```python
from build123d import *

# Parameters (mm, degrees)
EXTRUDE_1_DEPTH        = 25
HOLE_WIZARD_M4_1_D     = 3.3
HOLE_WIZARD_M4_1_DEPTH = 20
HOLE_WIZARD_M4_1_TIP   = 0.991420021
SKETCH_5_R             = 2
EXTRUDE_2_DEPTH        = 6


# Read off the part's stored shape, not the designer's step: M4 机械螺纹 螺柱1
with BuildPart() as part:
    # 草图1 → 凸台-拉伸1 (new body)
    with BuildSketch(Plane.XY):
        Polygon((-3.464101615, 0), (-1.732050808, -3), (1.732050808, -3), (3.464101615, 0), (1.732050808, 3), (-1.732050808, 3), align=None)
    extrude(amount=EXTRUDE_1_DEPTH)

    # M4 螺纹孔1
    with Locations(Plane.XY.offset(25)):
        with Locations((0, 0)):
            Hole(HOLE_WIZARD_M4_1_D / 2, depth=HOLE_WIZARD_M4_1_DEPTH)
            with Locations((0, 0, -(HOLE_WIZARD_M4_1_DEPTH + HOLE_WIZARD_M4_1_TIP / 2))):  # 118° drill point
                Cone(0, HOLE_WIZARD_M4_1_D / 2, HOLE_WIZARD_M4_1_TIP, mode=Mode.SUBTRACT)

    # 草图5 → 凸台-拉伸2 (add)
    with BuildSketch(Plane(origin=(0, 0, 0), x_dir=(-1, 0, 0), z_dir=(0, 0, -1))):
        Circle(SKETCH_5_R)
    extrude(amount=EXTRUDE_2_DEPTH)

    # M4 机械螺纹 螺柱1 outline → M4 机械螺纹 螺柱1 (revolve, cut)
    with BuildSketch(Plane.XZ):
        Polygon((2, -5.621), (1.621, -6), (2, -6), align=None)
    revolve(axis=Axis((0, 0, 0), (0, 0, 1)), mode=Mode.SUBTRACT)


solid = part.part
```
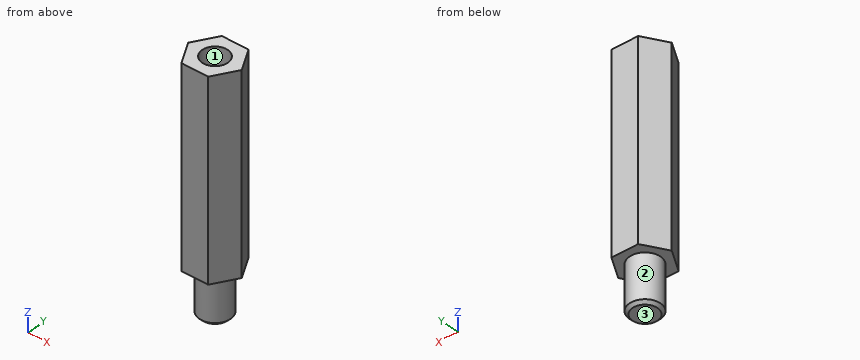
Could you check a few things on this model? Use its own coordinates, in mm. Face numbers are marked on the shaded views. Coordinates: 2 decimals unless noted, no trailing zeros. Write each loop counter-clockwise with the first axis right and the second up, starting at its lowest first coordinate (ties: lowest second). Pieces come first, ordered by that corner, then holes. Notation, with made-up numbers: M -27.5,54.5 L -5.5,54.5 A7 ccw -5.5,62.5 Z; hole C 68.5,19.25 d5. An arc over 180 degrees is marked long. Answer as CSV lines item,"result". Start each with the question number.
1) We'd pull the mould along Y, two halves only. Please class the marked faces 1, 2 and 3: +Y half, -Y half, draft (parallel to the pull), parting line (faces both ways), or undercut.
2) I want a section at A-A, the plane z = 16. Please give me the cut outline in (x, y).
3) For P1, Ø3, axis at y = 2.5, z = 10.5, coming from the -X side; P2, Ø2.5, axis at x = 0, y = 0, coming from the +Z side; P3, Ø3, axis at y = 1.5, z = -2, coming from the +X side, each with a flat end and sliding along its axis, tell me the tip position at first contact or that it passes through.
4) Please list where these lines run through material, in increasing order: line 1 (Y direction, x = 0, z = 15.5); line 2 (X direction, y = 0.5, z = 15.5); line 3 (Z direction, x = 1.75, y = 1.25). Write a range as from..to.
5) I want a section at B-B, the plane y = -2.5. Please give me the cut outline in (x, z).
Data:
1,face 1,"undercut"
1,face 2,"parting line"
1,face 3,"draft"
2,outline,"M -3.46,0 L -1.73,-3 L 1.73,-3 L 3.46,0 L 1.73,3 L -1.73,3 Z; hole C 0,0 d3.3"
3,P1,"stops at x = -2.89"
3,P2,"stops at z = 4.76"
3,P3,"stops at x = 2"
4,line 1,"y = -3..-1.65, 1.65..3"
4,line 2,"x = -3.18..-1.57, 1.57..3.18"
4,line 3,"z = 0..25"
5,outline,"M -2.02,0 L 2.02,0 L 2.02,25 L -2.02,25 Z"
